Source: CAD feature listing. Evaluate the final solid. Frame: model axes, mm. A direction names the side the tool comes from. Coordinates: 2 decimals unless noted, no trailing zeros. Loops run counter-clockwise (first coordinate to the right, second up) from the corner with the lowest first, then second, coordinate; pieces in that order, holes last.
Autodesk Fusion 360 part; units mm, degrees
sketch "Sketch1" plane through (0, 0, 0) normal (0, 0, 1) x (1, 0, 0)
  line L0 (0, 0) -> (7.4, 0) construction
  circle A0 centre (7.4, 0) radius 1.6
  line L1 (9, -4) -> (-9, -4)
  line L2 (-9, -4) -> (-9, 4)
  line L3 (-9, 4) -> (9, 4)
  line L4 (9, -4) -> (-9, 4) construction
  line L5 (-9, -4) -> (9, 4) construction
  line L6 (9, -4) -> (11, -4)
  line L7 (11, -4) -> (11, 4)
  line L8 (11, 4) -> (9, 4)
  line L9 (0, -4) -> (0, 4)
  dimension "d1" = 7.4
  dimension "d2" = 3.2
  dimension "d3" = 8
  dimension "d4" = 2
extrude "Extrude1" add sketch "Sketch1" along normal blind 2
extrude "Extrude2" add sketch "Sketch1" against normal blind 5 contours L1 L2 L3 L9
fillet "Fillet1" radius 1 4 edges at (11, -4, 1) (11, 4, 1) (-9, -4, -1.5) (-9, 4, -1.5)
sketch "Sketch2" plane through (0, -4, 0) normal (0, -1, 0) x (1, 0, 0)
  line L0 (-8, 2) -> (-8, -5)
  line L1 (-8, -5) -> (0, -5)
  line L2 (0, -5) -> (0, 0)
  line L3 (0, 0) -> (10, 0)
  line L4 (10, 0) -> (10, 2)
  line L5 (10, 2) -> (-8, 2)
  line L6 (-6.2, -1) -> (-3.2, -1)
  line L7 (-3.2, -1) -> (-3.2, -3)
  line L8 (-3.2, -3) -> (-6.2, -3)
  line L9 (-6.2, -3) -> (-6.2, -1)
  dimension "d11" = 3
  dimension "d12" = 2
extrude "Extrude3" cut sketch "Sketch2" against normal blind 8 contours L6 L7 L8 L9
sketch "Sketch3" plane through (0, -4, 0) normal (0, -1, 0) x (1, 0, 0)
  line L0 (-3.2, -1) -> (-3.2, -3)
  line L1 (-3.2, -3) -> (-6.2, -3)
  line L2 (-6.2, -3) -> (-6.2, -1)
  line L3 (-6.2, -1) -> (-3.2, -1)
  line L4 (-8, 2) -> (-8, -5)
  line L5 (-8, -5) -> (0, -5)
  line L6 (0, -5) -> (0, 0)
  line L7 (0, 0) -> (10, 0)
  line L8 (10, 0) -> (10, 2)
  line L9 (10, 2) -> (-8, 2)
  line L10 (-6.2, -1) -> (-3.2, -1)
  line L11 (-3.2, -1) -> (-3.2, 2)
  line L12 (-3.2, 2) -> (-6.2, 2)
  line L13 (-6.2, 2) -> (-6.2, -1)
extrude "Extrude4" cut sketch "Sketch3" against normal blind 1 contours L3 L9 L10 L11 L12 L13
fillet "Fillet3" radius 1 2 edges at (-6.2, -4, -0.5) (-3.2, -4, -0.5)
fillet "Fillet4" radius 1.75 2 edges at (-4.7, -3, -1) (-4.7, 4, -1)
fillet "Fillet2" [suppressed]
Q1. Section D-D, the plane z = -1.25. Return the cut outline in (x, y), plus the area to 3 significant figures.
Q2. Section C-C, the plane x = 7.4. Return the cut outline in (y, z).
Q3. Section A-A, the plane y = 0. Return the cut outline in (x, z).
Q4. Access query for faces 4 (the flat face through (0, 0, -2)), 5 (the flat face through (-5, -3, 1)), 6 (the flat face through (-5, 0, -1)). Directions: +Z, -Z, +X, -X, +Y, -Y. A direction counts if a zero-diameter tool reaches every point of the face in a straight line with its end or side. Return the directions, or none.
Q5. Line query: line 1 along Y through (x, z) = (7.4, 0.5); line 2 along X through (y, z) = (2, -2); line 3 along Z through (x, y) = (3.25, -0.75). Output: solid intervals per line, ascending.
Q6. Contact query for flat-ended pins moving along their axis: pin 1 Ø3 at (y, z) = (1, -3.5) entering from +X; pin 2 Ø0.6 at (x, z) = (-5, 1.5) entering from -Y; pin 3 Ø3 at (x, y) = (2, -1.5) entering from -Z. Output: stop coordinate, or through.
Q7. Draft query along Y for faces 1 (the cylindrical face through (-4.679, -2.501, -0.474)), 2 (the cylindrical face through (9, 0, 1)), 3 (the flat face through (11, 0, 1)). Return one class per face: +Y half, -Y half, draft (parallel to the pull), parting line (faces both ways), or undercut.
Derived:
1. outline: (-9, -3) arc R1 ccw to (-8, -4) - (-7.2, -4) arc R1 ccw to (-6.2, -3) - (-6.2, 4) - (-8, 4) arc R1 ccw to (-9, 3) - close; (-3.2, -3) arc R1 ccw to (-2.2, -4) - (0, -4) - (0, 4) - (-3.2, 4) - close
1. area: 47.1 mm2
2. outline: (-4, 0) - (-1.6, 0) - (-1.6, 2) - (-4, 2) - close; (1.6, 0) - (4, 0) - (4, 2) - (1.6, 2) - close
3. outline: (-9, -5) - (0, -5) - (0, 0) - (5.8, 0) - (5.8, 2) - (-9, 2) - close; (9, 0) - (11, 0) - (11, 2) - (9, 2) - close; hole (-6.2, -3) - (-3.2, -3) - (-3.2, -1) - (-6.2, -1) - close
4. face 4: -Z, +X, +Y, -Y
4. face 5: +Z, -Y
4. face 6: +Y, -Y
5. line 1: y = -4 to -1.6, 1.6 to 4
5. line 2: x = -9 to -6.2, -3.2 to 0
5. line 3: z = 0 to 2
6. pin 1: stops at x = 0
6. pin 2: stops at y = -3
6. pin 3: stops at z = 0
7. face 1: -Y half
7. face 2: undercut
7. face 3: draft
